Build history of the part. All positions in model axes, mm. A direction names the side the tool comes from. Coordinates: 2 decimals unless noted, no trailing zeros. Order: outer loops, then holes, each group sorted by start corner. A loop starts at its lowest first (then second) coordinate and runs counter-clockwise, first axis right, second up. Notation, with made-up numbers: (84, 9) - (93, 9) arc R25 cw to (93, 42) - close; hole circle Ø1 at (87, 55). An arc over 180 degrees is marked (long way). Write each question's results on one line, items separated by ' | '.
from build123d import *

# Parameters (mm, degrees)
SKETCH1_R           = 9
BOSS_EXTRUDE1_DEPTH = 3
SKETCH2_R           = 2.5
BOSS_EXTRUDE2_DEPTH = 10
BOSS_EXTRUDE3_DEPTH = 9


with BuildPart() as part:
    # Sketch1 → Boss-Extrude1 (new body)
    with BuildSketch(Plane(origin=(0, 0, 0), x_dir=(1, 0, 0), z_dir=(0, 1, 0))):
        Circle(SKETCH1_R)
    extrude(amount=BOSS_EXTRUDE1_DEPTH)

    # Sketch2 → Boss-Extrude2 (add)
    with BuildSketch(Plane(origin=(0, 3, 0), x_dir=(1, 0, 0), z_dir=(0, 1, 0))):
        with Locations((5, 0)):
            Circle(SKETCH2_R)
    extrude(amount=BOSS_EXTRUDE2_DEPTH)

    # Sketch3 → Boss-Extrude3 (add)
    with BuildSketch(Plane.XZ):
        Polygon((2.713546265, 0), (1.356773133, 2.35), (-1.356773133, 2.35), (-2.713546265, 0), (-1.356773133, -2.35), (1.356773133, -2.35), align=None)
    extrude(amount=BOSS_EXTRUDE3_DEPTH)


solid = part.part
1. Band-saw the part on B-B on y = -1. Give the cut face in (x, z).
Solved:
outline: (-2.71, 0) - (-1.36, -2.35) - (1.36, -2.35) - (2.71, 0) - (1.36, 2.35) - (-1.36, 2.35) - close
2. Probe line 1 (Y direction, x = 0, z = -0.25); line 2 (Y direction, x = 4.5, z = -3.5); line 3 (X direction, y = -7.25, z = -1). List the from-to ranges inside material, lowest first.
Solved:
line 1: y = -9 to 3 | line 2: y = 0 to 3 | line 3: x = -2.14 to 2.14
3. Band-saw the part on C-C on z = -1.5. Give the cut face in (x, y), then the cut area to 4 significant figures.
Solved:
outline: (-8.87, 0) - (-1.85, 0) - (-1.85, -9) - (1.85, -9) - (1.85, 0) - (8.87, 0) - (8.87, 3) - (7, 3) - (7, 13) - (3, 13) - (3, 3) - (-8.87, 3) - close | area: 126.5 mm2
4. Band-saw the part on A-A on x = 5. Give the cut face in (y, z), then the cut area to 3 significant figures.
Solved:
outline: (0, -7.48) - (3, -7.48) - (3, -2.5) - (13, -2.5) - (13, 2.5) - (3, 2.5) - (3, 7.48) - (0, 7.48) - close | area: 94.9 mm2
5. Tool access for faces 1 (the face through (2, 0, 2)), 2 (the face through (-2.045, -4.437, -1.159)), 3 (the face through (-2.026, -4.437, 1.191)), 4 (the face through (7.385, 7.93, -0.751)): list every direction of +Z, -Z, +X, -X, +Y, -Y with a clear straight run to the whole face (end or side of a thin tool).
Solved:
face 1: -Y | face 2: -Z, -X, -Y | face 3: +Z, -X, -Y | face 4: +Y
6. Band-saw the part on D-D on x = 0. Give the cut face in (y, z), then the cut area to 3 significant figures.
Solved:
outline: (-9, -2.35) - (0, -2.35) - (0, -9) - (3, -9) - (3, 9) - (0, 9) - (0, 2.35) - (-9, 2.35) - close | area: 96.3 mm2
7. Drop flat-ended pins along their axis: pin 1 Ø1 at (x, z) = (0.5, 6.5) entering from -Y; pin 2 Ø9 at (x, z) = (-2, 1) entering from +Y; pin 3 Ø4 at (x, z) = (2.5, 2) entering from +Y; pin 4 Ø0.8 at (x, y) = (0.5, -5) entering from +Z. Give the stop position or say it passes through.
Solved:
pin 1: stops at y = 0 | pin 2: stops at y = 3 | pin 3: stops at y = 13 | pin 4: stops at z = 2.35
